Part model, mm, in its own coordinate system. Give positions to 0.01 mm unless a question says otherwise; leave off trailing zeros. Order: outer loops, then holes, each group sorted by start corner. A loop starts at its lowest first (then second) coordinate and runs counter-clockwise, first axis right, second up. Notation, with made-up numbers: M 86.5,16 L 122.5,16 A21 cw 122.5,31 Z; hole C -33,18 d9. An arc over 180 degrees is marked long. Write each question's results on one line, items separated by ' | '. Start each with the question number.
Autodesk Inventor part; units mm, degrees
ref_plane "YZ Plane" through (0, 0, 0) normal (1, 0, 0) x (0, 1, 0)
ref_plane "XZ Plane" through (0, 0, 0) normal (0, 1, 0) x (-1, 0, 0)
ref_plane "XY Plane" through (0, 0, 0) normal (0, 0, 1) x (1, 0, 0)
sketch "Sketch1" plane through (0, 0, 0) normal (0, 0, 1) x (1, 0, 0)
  line L0 (-40, -7) -> (40, -7)
  line L1 (40, -7) -> (40, 7)
  line L2 (40, 7) -> (-40, 7)
  line L3 (-40, 7) -> (-40, -7)
  line L4 (-40, -7) -> (40, 7) construction
  line L5 (40, -7) -> (-40, 7) construction
  point P0 (0, 0)
  dimension "d0" = 80
  dimension "d1" = 14
extrude "Extrusion1" add sketch "Sketch1" along normal blind 1
sketch "Sketch2" plane through (0, 0, 1) normal (0, 0, 1) x (1, 0, 0)
  point P0 (0, 0)
  point P1 (0, 0)
hole "Hole1" at (0, 0, 1) direction (0, 0, -1) diameter 5.5 depth 8 tip angle 118
sketch "Sketch3" plane through (0, 0, 1) normal (0, 0, 1) x (1, 0, 0)
  line L0 (-34, 0) -> (34, 0) construction
  point P0 (0, 0)
  point P1 (0, 0)
  dimension "d11" = 68
hole "Hole2" at (-34, 0, 1) at (34, 0, 1) direction (0, 0, -1) diameter 5.5 depth 8 tip angle 118
properties part number "Cu_Cap" material "Copper"
(1) Probe L1, parallel to X at y = 0, z = 0.8; L2, parallel to X at y = -2.5, z = 0.3; L3, parallel to Y at x = 34, z = 0.35. List the from-to ranges inside material, lowest first.
(2) Saw through at A-A on x = 0. Give the cut face in (y, z).
(3) Saw through at C-C on z = 0.65. Give the cut face in (x, y), plus the area to 3 significant figures.
(4) Pull direction Y, two halves, no side cores. Call faces 1 (the cylindrical face through (31.273, 0.358, 0.493)), 2 (the flat face through (-1, 3, 0)): +Y half, -Y half, draft (parallel to the pull), parting line (faces both ways), or undercut.
(5) Saw through at B-B on y = -0.5. Give the cut face in (x, z).
(6) Saw through at D-D on x = 33. Give the cut face in (y, z), plus the area to 3 significant figures.
Taken from the geometry:
1) L1: x = -40 to -36.75, -31.25 to -2.75, 2.75 to 31.25, 36.75 to 40 | L2: x = -40 to -35.15, -32.85 to -1.15, 1.15 to 32.85, 35.15 to 40 | L3: y = -7 to -2.75, 2.75 to 7
2) outline: M -7,0 L -2.75,0 L -2.75,1 L -7,1 Z; M 2.75,0 L 7,0 L 7,1 L 2.75,1 Z
3) outline: M -40,-7 L 40,-7 L 40,7 L -40,7 Z; hole C -34,0 d5.5; hole C 0,0 d5.5; hole C 34,0 d5.5 | area: 1,050 mm²
4) face 1: undercut | face 2: draft
5) outline: M -40,0 L -36.7,0 L -36.7,1 L -40,1 Z; M -31.3,0 L -2.7,0 L -2.7,1 L -31.3,1 Z; M 2.7,0 L 31.3,0 L 31.3,1 L 2.7,1 Z; M 36.7,0 L 40,0 L 40,1 L 36.7,1 Z
6) outline: M -7,0 L -2.56,0 L -2.56,1 L -7,1 Z; M 2.56,0 L 7,0 L 7,1 L 2.56,1 Z | area: 8.88 mm²
